The model under review builds one solid part; all positions refer to its coordinate system, in mm. Face numbers are marked on the shaded views. A direction names the side the tool comes from. Give positions to 0.01 mm unless a question says otherwise; leave off trailing zeros. Write each loop counter-clockwise with the first axis right and the second up, starting at its lowest first coordinate (ties: lowest second). Pieces come first, ordered by that corner, then holes.
from build123d import *

# Parameters (mm, degrees)
F0_W     = 50
F0_H     = 100
F1_DEPTH = 50
F2_SIZE2 = 15
F2_SIZE  = 15
F4_D     = 15
F4_DEPTH = 15
F4_TIP   = 4.5064546427
F5_R     = 5
F6_R     = 5


with BuildPart() as f1:
    # F0 (on Top) → F1 (new body)
    with BuildSketch(Plane.XY):
        with Locations((25, 50)):
            Rectangle(F0_W, F0_H)
    extrude(amount=F1_DEPTH)

    # F2
    f2_edges = [f1.edges().sort_by_distance(p)[0] for p in [
        (50, 50, 50),
    ]]
    chamfer(f2_edges, length=F2_SIZE, length2=F2_SIZE2)

    # F4
    with Locations(Plane(origin=(42.5, 0, 42.5), x_dir=(0, 1, 0), z_dir=(0.7071067812, 0, 0.7071067812))):
        with Locations((30, 0), (70, 0)):
            Hole(F4_D / 2, depth=F4_DEPTH)
            with Locations((0, 0, -(F4_DEPTH + F4_TIP / 2))):  # 118° drill point
                Cone(0, F4_D / 2, F4_TIP, mode=Mode.SUBTRACT)

    # F5
    f5_edges = [f1.edges().sort_by_distance(p)[0] for p in [
        (0, 100, 25),
    ]]
    fillet(f5_edges, radius=F5_R)

    # F6
    f6_edges = [f1.edges().sort_by_distance(p)[0] for p in [
        (0, 0, 25),
    ]]
    fillet(f6_edges, radius=F6_R)


solid = f1.part
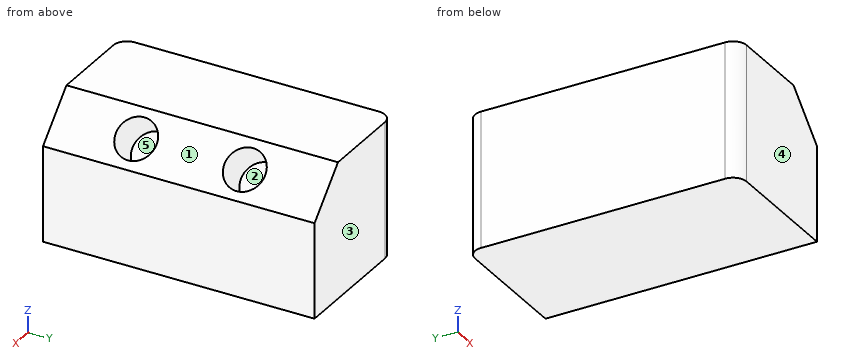
1) Consider section B-B, the plane z = 33.5. State how many separate pieces and enclosed holes the cut face has, then the cut area to 3 significant figures.
2) Tool access review of the marked faces 4 and 5: name each direction out of +Z, -Z, +X, -X, +Y, -Y from which nothing blocks a thin tool from reaching the whole face with its end or side.
3) Consider section A-A, the plane y = 80. Give the boundary of the cut face in (x, z), then the cut area to 3 significant figures.
4) To check wall thickness, follow probe 1 along X at (y, z) = (66.5, 47.5); probe 2 along X at (y, z) = (74, 30); probe 3 along Y at (x, z) = (4, 22). State the ranges of each line that lie inside material, in increasing order.
5) The part is to be moulded in two halves that separate along Y. For the marked faces 1, 2 and 3, say which applies: +Y half, -Y half, draft (parallel to the pull), parting line (faces both ways), or undercut.
Answer block:
1. separate pieces: 1
1. enclosed holes: 2
1. area: 4,590 mm2
2. face 4: +Z, -Z, +X, -X, -Y
2. face 5: none
3. outline: (0, 0) - (50, 0) - (50, 35) - (35, 50) - (0, 50) - close
3. area: 2,390 mm2
4. probe 1: x = 0 to 37.5
4. probe 2: x = 0 to 30.85, 38.97 to 50
4. probe 3: y = 0.1 to 99.9
5. face 1: draft
5. face 2: undercut
5. face 3: +Y half
